Design review of the part built by this model. Coordinates are the model's own, in mm. A direction names the side the tool comes from. Give positions to 0.01 mm unless a question says otherwise; leave off trailing zeros. Order: outer loops, then holes, each group sorted by start corner. A loop starts at its lowest first (then second) coordinate and runs counter-clockwise, first axis right, second up. Notation, with made-up numbers: (42.25, 73.5) -> (52.25, 73.5) arc R24 cw to (52.25, 86.5) -> close; hole circle Ø4 at (52.5, 67.25). An arc over 180 degrees is marked (long way). One line per item, written item: value.
from build123d import *

# Parameters (mm, degrees)
ESQUISSE2_R             = 25
BOSS_EXTRU_1_DEPTH      = 35
ESQUISSE3_R             = 10
ENL_V_MAT_EXTRU_1_DEPTH = 35
TROU_TARAUD_M62_D       = 5
TROU_TARAUD_M62_DEPTH   = 20
TROU_TARAUD_M62_TIP     = 1.502151548


with BuildPart() as part:
    # Esquisse2 → Boss.-Extru.1 (new body)
    with BuildSketch(Plane(origin=(0, 0, 0), x_dir=(1, 0, 0), z_dir=(0, 1, 0))):
        with Locations(Location((0, 0, 0), (0, 0, 270))):  # turned: the seam where the file's is
            Circle(ESQUISSE2_R)
    extrude(amount=BOSS_EXTRU_1_DEPTH)

    # Esquisse3 → Enlèv. mat.-Extru.1 (cut)
    with BuildSketch(Plane(origin=(0, 35, 0), x_dir=(1, 0, 0), z_dir=(0, 1, 0))):
        with Locations(Location((0, 0, 0), (0, 0, 270))):  # turned: the seam where the file's is
            Circle(ESQUISSE3_R)
    extrude(amount=-ENL_V_MAT_EXTRU_1_DEPTH, mode=Mode.SUBTRACT)

    # Trou taraudé M62
    with Locations(Plane(origin=(0, 0, 0), x_dir=(-1, 0, 0), z_dir=(0, -1, 0))):
        with Locations((17.5, 0), (-8.74846, -15.156333581), (-8.753079729, 15.153666067)):
            Hole(TROU_TARAUD_M62_D / 2, depth=TROU_TARAUD_M62_DEPTH)
            with Locations((0, 0, -(TROU_TARAUD_M62_DEPTH + TROU_TARAUD_M62_TIP / 2))):  # 118° drill point
                Cone(0, TROU_TARAUD_M62_D / 2, TROU_TARAUD_M62_TIP, mode=Mode.SUBTRACT)


solid = part.part
Item 1: Machinability: for faces 1 (the cylindrical face through (-20, 10, 0)), 2 (the cylindrical face through (-9.76, 17.74, -2.17)), which of the approach directions +Z, -Z, +X, -X, +Y, -Y give a long, thin tool a straight path to every point of the face, cutting with its end or side? Answer none if there is none.
Returned:
face 1: -Y
face 2: +Y, -Y
Item 2: Add section B-B on y = 15. Give the boundary of the cut face in (x, z), plus the area to 3 significant figures.
Returned:
outline: circle Ø50 at (0, 0); hole circle Ø5 at (-17.5, 0); hole circle Ø20 at (0, 0); hole circle Ø5 at (8.75, -15.15); hole circle Ø5 at (8.75, 15.16)
area: 1,590 mm²
Item 3: Add section A-A on x = 0. Give the boundary of the cut face in (y, z).
Returned:
outline: (0, -25) -> (35, -25) -> (35, -10) -> (0, -10) -> close; (0, 10) -> (35, 10) -> (35, 25) -> (0, 25) -> close
Item 4: To check wall thickness, follow line 1 along X through (y, z) = (27.5, -0.5) (1 decimal); line 2 along Z through (x, y) = (7, 16.5); line 3 along X through (y, z) = (6, 14.5). State the ranges of each line that lie inside material, in increasing order. Write a range as from..to.
Returned:
line 1: -25..-10, 10..25
line 2: -24..-16.94, -13.37..-7.14, 7.14..13.37, 16.94..24
line 3: -20.37..6.34, 11.16..20.37
Item 5: Draft analysis for pull direction X (two halves, no side actions). For faces 3 (the flat face through (0, 0, 11)), 4 (the conical face through (-17.155, 21.241, 0.264)), 5 (the cylindrical face through (7.509, 17.255, 23.846)), state which applies: pulls with the +X half, pulls with the -X half, needs draft (parallel to the pull), parting line crosses it, or undercut.
Returned:
face 3: needs draft
face 4: undercut
face 5: parting line crosses it
Item 6: Add section C-C on x = -7. Give the boundary of the cut face in (y, z), plus the area to 3 significant figures.
Returned:
outline: (0, -24) -> (35, -24) -> (35, -7.14) -> (0, -7.14) -> close; (0, 7.14) -> (35, 7.14) -> (35, 24) -> (0, 24) -> close
area: 1,180 mm²
Item 7: Add section D-D on y = 27. Give the boundary of the cut face in (x, z), plus the area to 3 significant figures.
Returned:
outline: circle Ø50 at (0, 0); hole circle Ø20 at (0, 0)
area: 1,650 mm²
Item 8: Clearance check with flat-ended pins moving along their axes: P1, Ø2, axis at x = -11.5, y = 22, coming from the +Z side; P2, Ø4, axis at x = -17.5, z = 0, coming from the -Y side; P3, Ø12, axis at x = -15.5, y = 11, coming from the -Z side. State where each tip first meets the part, or that it passes through.
Returned:
P1: z = 22.69
P2: y = 20.3
P3: z = -23.12
